from build123d import *

# Parameters (mm, degrees)
EXTRUDE_1_DEPTH            = 2
SKETCH_2_W                 = 22.014506199136
SKETCH_2_H                 = 16
EXTRUDE_2_DEPTH            = 15
CUT_EXTRUDE_1_REACH        = 27.171
SKETCH_3_R                 = 1.0000000000000016
CUT_EXTRUDE_2_DEPTH        = 1
PATTERN_LINEAR_1_COUNT     = 3
PATTERN_LINEAR_1_PITCH     = 2
PATTERN_LINEAR_1_COL_COUNT = 3
PATTERN_LINEAR_1_COL_PITCH = 2
CUT_EXTRUDE_3_DEPTH        = 5
FILLET_4_R                 = 2
CUT_EXTRUDE_5_DEPTH        = 15
MIRROR_3_COPY_1_DEPTH      = 15
FILLET_6_R                 = 0.2
FILLET_7_R                 = 2


with BuildPart() as part:
    # 草图1 → 凸台-拉伸1 (new body)
    with BuildSketch(Plane(origin=(0, 0, 0), x_dir=(1, 0, 0), z_dir=(0, 1, 0))):
        with BuildLine():
            Line((-16.75, -4.000000000000002), (-16.75, 3.9999999999999982))
            Line((-16.75, 3.9999999999999982), (-11.51489754486675, 7.641810403570972))
            ThreePointArc((-11.51489754486675, 7.641810403570972), (-10.971257997306036, 7.908352798507383), (-10.372768568469548, 7.9999999999999964))
            Line((-10.372768568469548, 7.9999999999999964), (10.372768568469544, 8))
            ThreePointArc((10.372768568469544, 8), (10.971257997306031, 7.908352798507387), (11.514897544866734, 7.641810403570965))
            Line((11.514897544866734, 7.641810403570965), (16.75, 4.000000000000005))
            Line((16.75, 4.000000000000005), (16.75, -3.9999999999999947))
            Line((16.75, -3.9999999999999947), (11.514897544866738, -7.641810403570964))
            ThreePointArc((11.514897544866738, -7.641810403570964), (10.971257997306049, -7.908352798507378), (10.37276856846958, -7.9999999999999964))
            Line((10.37276856846958, -7.9999999999999964), (-10.372768568469548, -7.999999999999998))
            ThreePointArc((-10.372768568469548, -7.999999999999998), (-10.971257997306035, -7.908352798507385), (-11.51489754486674, -7.641810403570962))
            Line((-11.51489754486674, -7.641810403570962), (-16.75, -4.000000000000002))
        make_face()
    extrude(amount=EXTRUDE_1_DEPTH)

    # 草图2 → 凸台-拉伸2 (add)
    with BuildSketch(Plane(origin=(0, 2, 0), x_dir=(1, 0, 0), z_dir=(0, 1, 0))):
        Rectangle(SKETCH_2_W, SKETCH_2_H)
    extrude(amount=EXTRUDE_2_DEPTH)

    # 草图3 → 切除-拉伸1 (cut, up to next)
    with BuildSketch(Plane.XZ, mode=Mode.PRIVATE) as cut_extrude_1_sk1:
        with Locations(Location((-12.5, -1.53e-15, 0), (0, 0, 270))):
            Circle(SKETCH_3_R)
    cut_extrude_1_tool1 = extrude(cut_extrude_1_sk1.sketch, amount=-CUT_EXTRUDE_1_REACH, mode=Mode.PRIVATE) & part.part
    cut_extrude_1 = cut_extrude_1_tool1.solids().sort_by_distance((-12.5, 0, 0))[0]
    add(cut_extrude_1, mode=Mode.SUBTRACT)

    # 镜向1: 切除-拉伸1 across plane
    add(cut_extrude_1.mirror(Plane(origin=(0, 0, 0), x_dir=(0, 0, 1), z_dir=(1, 0, 0))), mode=Mode.SUBTRACT)

    # 草图4 → 切除-拉伸2 (cut)
    with BuildSketch(Plane(origin=(0, 17, 0), x_dir=(1, 0, 0), z_dir=(0, 1, 0))):
        Polygon((0, 0.5), (7, 0.5), (7, -0.5), (0, -0.5), (-7, -0.5), (-7, 0.5), align=None)
    cut_extrude_2 = extrude(amount=-CUT_EXTRUDE_2_DEPTH, mode=Mode.SUBTRACT)

    # 阵列(线性)1: 切除-拉伸2 ×3
    with Locations(*[(0, 0, i * PATTERN_LINEAR_1_PITCH) for i in range(1, PATTERN_LINEAR_1_COUNT)]):
        add(cut_extrude_2, mode=Mode.SUBTRACT)

    # 阵列(线性)1 col: 切除-拉伸2 ×3
    with Locations(*[(0, 0, -i * PATTERN_LINEAR_1_COL_PITCH) for i in range(1, PATTERN_LINEAR_1_COL_COUNT)]):
        add(cut_extrude_2, mode=Mode.SUBTRACT)

    # 草图5 → 切除-拉伸3 (cut)
    with BuildSketch(Plane(origin=(0, 16, 0), x_dir=(1, 0, 0), z_dir=(0, 1, 0))):
        Polygon((9, 6.0000000000000036), (9.000000000000002, -5.999999999999997), (-8.999999999999998, -6.000000000000001), (-8.999999999999998, 5.999999999999999), align=None)
    extrude(amount=-CUT_EXTRUDE_3_DEPTH, mode=Mode.SUBTRACT)

    # 圆角4
    fillet_4_edges = [part.edges().sort_by_distance(p)[0] for p in [
        (-16.75, 1, 4.000000000000002),
        (-16.75, 1, -3.9999999999999982),
        (16.75, 1, -4.000000000000005),
        (16.75, 1, 3.9999999999999947),
    ]]
    fillet(fillet_4_edges, radius=FILLET_4_R)

    # 草图8 → 切除-拉伸5 (cut)
    with BuildSketch(Plane(origin=(0, 17, 0), x_dir=(1, 0, 0), z_dir=(0, 1, 0))):
        with BuildLine():
            Line((-9.007253099567999, 8), (-11.007253099568, 8))
            Line((-11.007253099568, 8), (-11.007253099568, 6))
            ThreePointArc((-11.007253099568, 6), (-10.421466661941093, 7.414213562373095), (-9.007253099567999, 8))
        make_face()
    cut_extrude_5 = extrude(amount=-CUT_EXTRUDE_5_DEPTH, mode=Mode.SUBTRACT)

    # 镜向2: 切除-拉伸5 across plane
    add(cut_extrude_5.mirror(Plane(origin=(0, 0, 0), x_dir=(0, 0, 1), z_dir=(1, 0, 0))), mode=Mode.SUBTRACT)

    # 镜向3: 切除-拉伸5 across plane
    add(cut_extrude_5.mirror(Plane.XY), mode=Mode.SUBTRACT)

    # 镜向3 copy 1 sketch → 镜向3 copy 1 (cut)
    with BuildSketch(Plane(origin=(0, 17, 0), x_dir=(-1, 0, 0), z_dir=(0, 1, 0))):
        with BuildLine():
            Line((-9.007253099567999, 8), (-11.007253099568, 8))
            Line((-11.007253099568, 8), (-11.007253099568, 6))
            ThreePointArc((-11.007253099568, 6), (-10.421466661941093, 7.414213562373095), (-9.007253099567999, 8))
        make_face()
    extrude(amount=-MIRROR_3_COPY_1_DEPTH, mode=Mode.SUBTRACT)

    # 圆角6
    fillet_6_edges = [part.edges().sort_by_distance(p)[0] for p in [
        (10.971257997306049, 2, 7.908352798507378),
        (13.703513260631969, 2, 6.119295123038627),
        (-16.75, 2, -8.9e-16),
        (-13.70351326063197, 2, 6.119295123038629),
        (-16.522605138319644, 2, 3.881182710057475),
        (-16.522605138319644, 2, -3.881182710057476),
        (13.703513260631965, 2, -6.119295123038633),
        (16.75, 2, -3.55e-15),
        (16.522605138319644, 2, 3.8811827100574723),
        (16.52260513831964, 2, -3.8811827100574794),
        (-9.690010834018773, 2, -8),
        (9.690010834018771, 2, -8),
        (-9.690010834018773, 2, 8),
        (9.69001083401879, 2, 8),
        (10.97125799730603, 2, -7.908352798507387),
        (-10.971257997306036, 2, -7.908352798507383),
        (-13.703513260631976, 2, -6.119295123038633),
        (-10.971257997306035, 2, 7.908352798507385),
    ]]
    fillet(fillet_6_edges, radius=FILLET_6_R)

    # 圆角7
    fillet_7_edges = [part.edges().sort_by_distance(p)[0] for p in [
        (-11.007253099568, 17, 0),
        (-10.421466661941095, 17, -7.414213562373094),
        (1.78e-15, 17, -8),
        (10.421466661941095, 17, -7.414213562373094),
        (-1.78e-15, 17, 8),
        (-10.421466661941095, 17, 7.414213562373094),
        (11.007253099568, 17, 0),
        (10.421466661941095, 17, 7.414213562373094),
    ]]
    fillet(fillet_7_edges, radius=FILLET_7_R)


solid = part.part
The listing builds one solid part. Answer for the finished solid, in the listing's coordinates (mm). A direction names the side the tool comes from. Coordinates: 2 decimals unless noted, no trailing zeros. Loops run counter-clockwise (first coordinate to the right, second up) from the corner with the lowest first, then second, coordinate; pieces in that order, holes last. Notation, with made-up numbers: (3, 20) -> (23, 20) arc R19 cw to (23, 54) -> close; hole circle Ø6 at (26, 15). An arc over 180 degrees is marked (long way). Write item = value, one per line. Start each with the question number.
1) Straight lines are drawn through the part: line 1 (X direction, y = 1.2, z = 0); line 2 (Y direction, x = 1, z = 3.25); line 3 (X direction, y = 14.75, z = 1.5). For each, find the intervals that lie inside material, in ascending order. Write a range as from..to.
2) Given pin 1 Ø0.8 at (x, y) = (0.5, 16.5) entering from +Z; pin 2 Ø4 at (x, y) = (-11.5, 6.5) entering from +Z; pin 3 Ø1.1 at (x, y) = (-3.5, 16.5) entering from -Z, each flat-ended and moving along its own axis, determine where each tip first touches the part or whether it passes through.
3) The mould has two halves that part along Y. Classify faces 1 (the face through (0, 14, 6)), 2 (the face through (-0.1, 16.5, -3.5)), 3 (the face through (0, 11, 0)): released by +Y, released by -Y, zero draft, split by the parting line, or undercut.
4) A cutting plane is placed at C-C (y = 5.75). Give the vertices of the cut face in (x, z), then the cut area to 3 significant figures.
5) A cutting plane is placed at B-B (x = -6.5). Count the separate pieces of the cut face and the enclosed holes in it, then the cut area to 3 significant figures.
6) A cutting plane is placed at A-A (z = 0). Give the vertices of the cut face in (x, y).
7) A tool of negligible diameter and unlimited length cuts with its end or side. For faces 4 (the face through (-10.437, 8.492, -7.399)), 5 (the face through (11.007, 8, 0)), 6 (the face through (-7, 16.5, 2)), 7 (the face through (0, 14, -6)), from which of +Z, -Z, +X, -X, +Y, -Y can it reach the whole face along a straight path? Write none if from no direction.
Responses:
q1.line_1 = -16.75..-13.5, -11.5..11.5, 13.5..16.75
q1.line_2 = 0..11, 16..17
q1.line_3 = -11.01..-9, 9..11.01
q2.pin_1 = 7.67
q2.pin_2 = 7.94
q2.pin_3 = -7.76
q3.face_1 = undercut
q3.face_2 = zero draft
q3.face_3 = undercut
q4.outline = (-11.01, -6) arc R2 ccw to (-9.01, -8) -> (9.01, -8) arc R2 ccw to (11.01, -6) -> (11.01, 6) arc R2 ccw to (9.01, 8) -> (-9.01, 8) arc R2 ccw to (-11.01, 6) -> close
q4.area = 349 mm²
q5.separate_pieces = 5
q5.enclosed_holes = 0
q5.area = 205 mm²
q6.outline = (-16.75, 0) -> (-13.5, 0) -> (-13.5, 2) -> (-16.55, 2) arc R0.2 ccw to (-16.75, 1.8) -> close; (-11.5, 0) -> (11.5, 0) -> (11.5, 2) -> (11.01, 2) -> (11.01, 15) arc R2 ccw to (9.01, 17) -> (7, 17) -> (7, 16) -> (9, 16) -> (9, 11) -> (-9, 11) -> (-9, 16) -> (-7, 16) -> (-7, 17) -> (-9.01, 17) arc R2 ccw to (-11.01, 15) -> (-11.01, 2) -> (-11.5, 2) -> close; (13.5, 0) -> (16.75, 0) -> (16.75, 1.8) arc R0.2 ccw to (16.55, 2) -> (13.5, 2) -> close
q7.face_4 = -Z, -X, +Y
q7.face_5 = +Z, -Z, +X, +Y
q7.face_6 = +Y
q7.face_7 = none
